CAD build for the part. Positions are in the model's coordinates, mm. Face numbers are marked on the shaded views. A direction names the side the tool comes from. Coordinates: 2 decimals unless noted, no trailing zeros. Order: outer loops, then holes, each group sorted by start corner. A loop starts at its lowest first (then second) coordinate and runs counter-clockwise, first axis right, second up. Notation, with made-up numbers: (17, 83) - (35, 83) arc R32 ccw to (35, 119) - close; hole circle Ø8 at (52.5, 89.25). An arc over 180 degrees is marked (long way). Use one line per item in the form item = value.
```python
from build123d import *

# Parameters (mm, degrees)
BOSS_EXTRUDE1_DEPTH = 9
SKETCH2_R           = 4.5
CUT_EXTRUDE1_DEPTH  = 152.052970841
CUT_EXTRUDE2_START  = 7
SKETCH3_R           = 8
CUT_EXTRUDE2_DEPTH  = 145.052970841
SKETCH4_R           = 2.75
CUT_EXTRUDE3_DEPTH  = 152.052970841


with BuildPart() as part:
    # Sketch1 → Boss-Extrude1 (new, symmetric)
    with BuildSketch(Plane.XY):
        with BuildLine():
            Line((0, 0), (0, 140))
            Line((0, 140), (2, 140))
            ThreePointArc((2, 140), (4.828427125, 138.828427125), (6, 136))
            Line((6, 136), (6, 14.039757872))
            ThreePointArc((6, 14.039757872), (7.050890653, 11.337397042), (9.651377029, 10.05497908))
            Line((9.651377029, 10.05497908), (52.348622971, 6.319454096))
            ThreePointArc((52.348622971, 6.319454096), (54.949109347, 5.037036134), (56, 2.334675304))
            Line((56, 2.334675304), (56, 0))
            Line((56, 0), (0, 0))
        make_face()
    extrude(amount=BOSS_EXTRUDE1_DEPTH, both=True)

    # Sketch2 → Cut-Extrude1 (cut, through all)
    with BuildSketch(Plane(origin=(0, 0, 0), x_dir=(1, 0, 0), z_dir=(0, 1, 0))):
        with Locations((36, 0)):
            Circle(SKETCH2_R)
    extrude(amount=CUT_EXTRUDE1_DEPTH, mode=Mode.SUBTRACT)

    # Sketch3 → Cut-Extrude2 (cut, through all)
    with BuildSketch(Plane(origin=(0, 0, 0), x_dir=(1, 0, 0), z_dir=(0, 1, 0)).offset(CUT_EXTRUDE2_START)):
        with Locations((36, 0)):
            Circle(SKETCH3_R)
    extrude(amount=CUT_EXTRUDE2_DEPTH, mode=Mode.SUBTRACT)

    # Sketch4 → Cut-Extrude3 (cut, through all)
    with BuildSketch(Plane(origin=(0, 0, 0), x_dir=(0, 0, -1), z_dir=(1, 0, 0))):
        with Locations(Location((0, 80, 0), (0, 0, 270))):
            Circle(SKETCH4_R)
        with Locations(Location((0, 120, 0), (0, 0, 270))):
            Circle(SKETCH4_R)
    extrude(amount=CUT_EXTRUDE3_DEPTH, mode=Mode.SUBTRACT)


solid = part.part
```
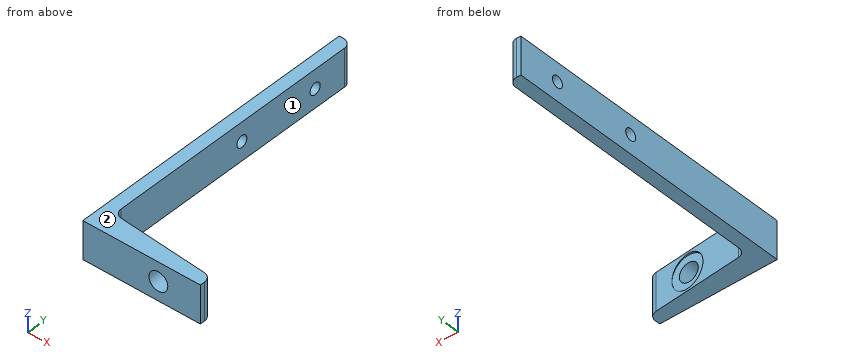
Item 1: Drill centre lines: line 1 (Z direction, x = 2, y = 120); line 2 (Z direction, x = 36, y = 1); line 3 (X direction, y = 41, z = 1). Where is each one in solid material? Low to high. Write a range as [from, to].
Derived:
line_1 = [-9, -2.75], [2.75, 9]
line_2 = [-9, -4.5], [4.5, 9]
line_3 = [0, 6]
Item 2: Cut at B-B, the plane z = 0. Write the cut outline in (x, y), plus the area to 3 significant figures.
Derived:
outline = (0, 0) - (31.5, 0) - (31.5, 7) - (28, 7) - (28, 8.45) - (9.65, 10.05) arc R4 cw to (6, 14.04) - (6, 77.25) - (0, 77.25) - close; (0, 82.75) - (6, 82.75) - (6, 117.25) - (0, 117.25) - close; (0, 122.75) - (6, 122.75) - (6, 136) arc R4 ccw to (2, 140) - (0, 140) - close; (40.5, 0) - (56, 0) - (56, 2.33) arc R4 ccw to (52.35, 6.32) - (44, 7.05) - (44, 7) - (40.5, 7) - close
area = 1,100 mm²
Item 3: Cut at C-C, the plane x = 36. Write the cut outline in (y, z), plus the area to 3 significant figures.
Derived:
outline = (0, -9) - (7.75, -9) - (7.75, -8) - (7, -8) - (7, -4.5) - (0, -4.5) - close; (0, 4.5) - (7, 4.5) - (7, 8) - (7.75, 8) - (7.75, 9) - (0, 9) - close
area = 64.5 mm²
Item 4: 3-axis set-ups, long thin cutter, end or side, ignore diameter. For the marked faces 1 and 2: which of +Z, -Z, +X, -X, +Y, -Y reach the whole face in a straight line?
Derived:
face_1 = +Z, -Z, +X, +Y
face_2 = +Z, +X, -X, +Y, -Y
Item 5: Cut at D-D, the plane y = 63. Write the cut outline in (x, z).
Derived:
outline = (0, -9) - (6, -9) - (6, 9) - (0, 9) - close
Item 6: Cut at A-A, the plane y = 80. Write the cut outline in (x, z).
Derived:
outline = (0, -9) - (6, -9) - (6, -2.75) - (0, -2.75) - close; (0, 2.75) - (6, 2.75) - (6, 9) - (0, 9) - close
Item 7: Drop flat-ended pins along their axis: pin 1 (10 mm diameter, centred on y = 74.5, z = -0.5, fed in from +X); pin 2 (4.5 mm diameter, centred on y = 80, z = 0, fed in from -X); pin 3 (8 mm diameter, centred on x = 28.5, z = -6.5, fed in from +Y); pin 4 (10.5 mm diameter, centred on x = 36, z = 0, fed in from -Y). Give the stop position or say it passes through.
Derived:
pin_1 = 6
pin_2 = through
pin_3 = 8.76
pin_4 = 0
